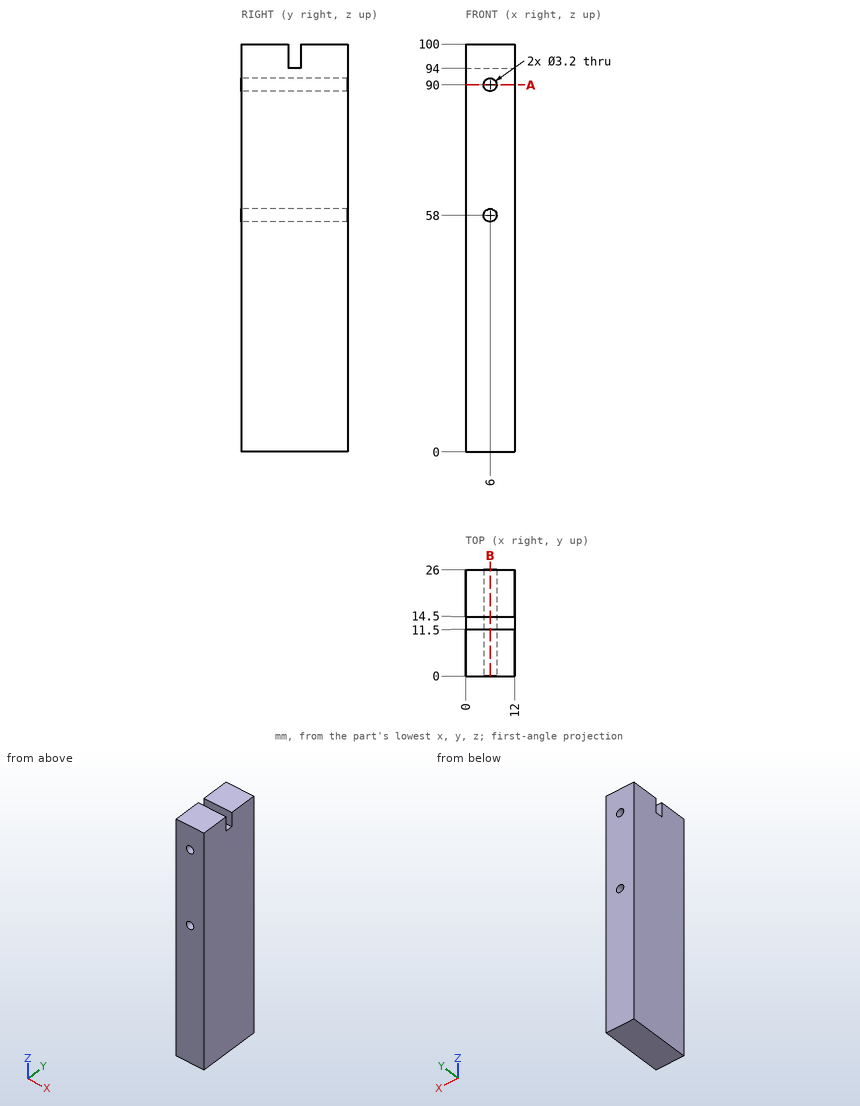
Could you check a few things on this drawing? It's one solid part, dimensions in mm from its lowest x, y, z. Give positions to 0.01 mm unless a question says otherwise; leave off trailing zeros. Write each loop counter-clockwise with the first axis right and the second up, starting at its lowest first coordinate (ties: lowest second). Pieces come first, ordered by that corner, then holes.
(1) If I drill on L1, parallel to X at y = 14.75, z = 90; L2, parallel to Z at x = 6.75, y = 7; L3, parallel to Z at x = 7, y = 8.25, over which ranges is the centre line in solid material (lowest first)?
Output values:
L1: x = 0 to 4.4, 7.6 to 12
L2: z = 0 to 56.59, 59.41 to 88.59, 91.41 to 100
L3: z = 0 to 56.75, 59.25 to 88.75, 91.25 to 100
(2) Will these pins go through, and if not, where does the flat tip stop? pin 1 (3 mm diameter, centred on x = 6, z = 90, fed in from +Y); pin 2 (1.5 mm diameter, centred on x = 4.5, y = 12.5, fed in from +Z).
Output values:
pin 1: passes through
pin 2: stops at z = 94
(3) Imagine slicing it at B-B, the plane x = 6. Write out the boundary of the cut face in (y, z), and give its area (3 significant figures).
Output values:
outline: (0, 0) - (26, 0) - (26, 56.4) - (0, 56.4) - close; (0, 59.6) - (26, 59.6) - (26, 88.4) - (0, 88.4) - close; (0, 91.6) - (26, 91.6) - (26, 100) - (14.5, 100) - (14.5, 94) - (11.5, 94) - (11.5, 100) - (0, 100) - close
area: 2,420 mm2
(4) Imagine slicing it at A-A, the plane z = 90. Write out the boundary of the cut face in (x, y).
Output values:
outline: (0, 0) - (4.4, 0) - (4.4, 26) - (0, 26) - close; (7.6, 0) - (12, 0) - (12, 26) - (7.6, 26) - close
